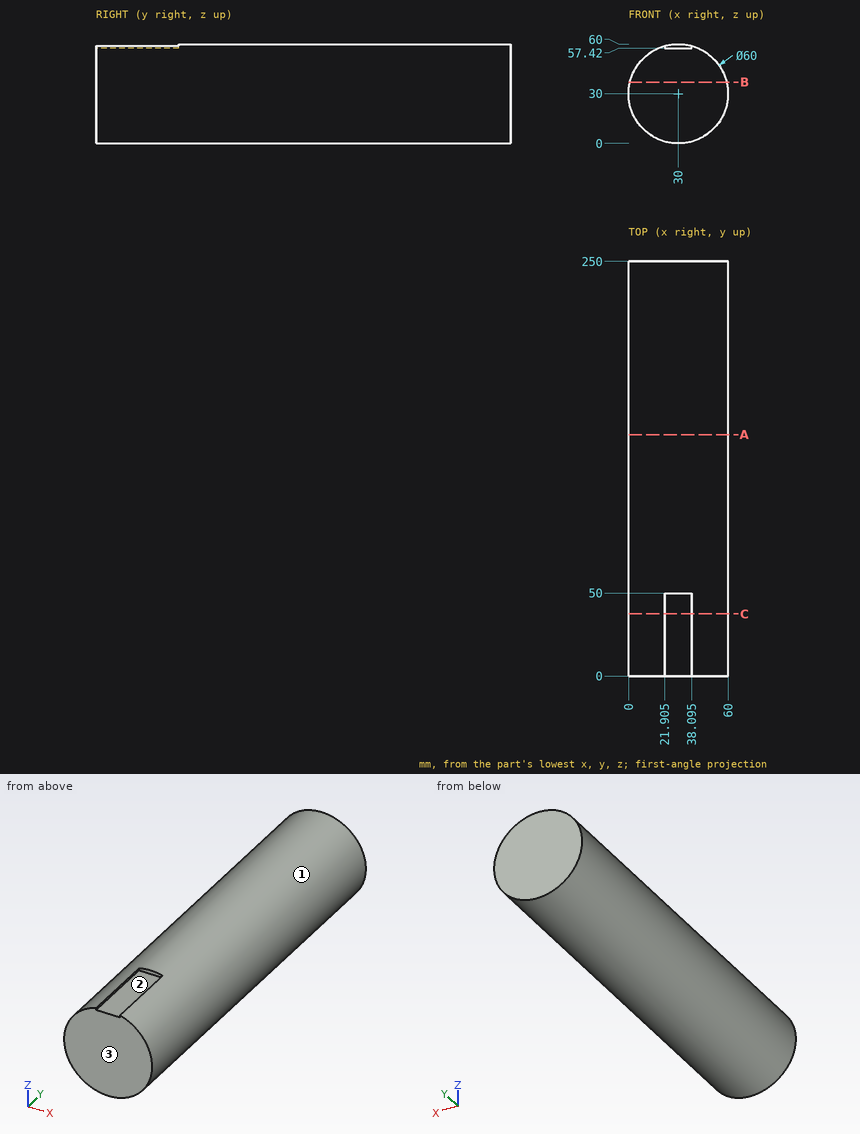
Geometry check sheet. Reference: drawing and pictorial views, mm from the part's lowest x, y, z. Round coordinates to 2 decimals unless told otherwise and drop trailing zeros. Write each loop counter-clockwise with the first axis right and the second up, starting at its lowest first coordinate (ties: lowest second). Pieces come first, ordered by that corner, then holes. Notation, with made-up numbers: (-14.5, 47) -> (27.5, 47) arc R33 cw to (27.5, 75) -> close; hole circle Ø5 at (59, 27). An arc over 180 degrees is marked (long way). One line per question, with ' | ' between items. Start each with the question number.
1. Scan lines: line 1 along X through (y, z) = (144.5, 30); line 2 along X through (y, z) = (219, 54.5) (1 decimal); line 3 along Z through (x, y) = (35.5, 190). Record each from-to range of solid material in increasing order. Write a range as from..to.
2. Sectioned sample at B-B, the plane z = 37. Record the cut outline in (x, y).
3. Sectioned sample at C-C, the plane y = 37.5. Record the cut outline in (x, z) (1 decimal).
4. Depth check by flat-ended pin: pin 1 (5 mm diameter, centred on x = 28.5, y = 16.5, fed in from +Z); pin 2 (8 mm diameter, centred on x = 52.5, z = 46.5, fed in from -Y); pin 3 (1.6 mm diameter, centred on y = 36.5, z = 58, fed in from -X) (1 decimal); pin 4 (4 mm diameter, centred on x = 20, y = 175, fed in from +Z). Enter the tip coordinate at first touch or a pass-through.
5. Release check for a two-part mould opening along X. For the marked faces 1, 2 and 3 record: +X half, -X half, draft (parallel to the pull), parting line (faces both ways), or undercut.
6. Sectioned sample at A-A, the plane y = 145.5. Record the cut outline in (x, z).
Taken from the geometry:
1) line 1: x = 0..60 | line 2: x = 12.7..47.3 | line 3: z = 0.51..59.49
2) outline: (0.83, 0) -> (59.17, 0) -> (59.17, 250) -> (0.83, 250) -> close
3) outline: (21.9, 57.4) -> (21.9, 58.9) arc R30 ccw (long way) to (38.1, 58.9) -> (38.1, 57.4) -> close
4) pin 1: stops at z = 57.42 | pin 2: stops at y = 0 | pin 3: stops at x = 17.3 | pin 4: stops at z = 58.91
5) face 1: parting line | face 2: undercut | face 3: draft
6) outline: circle Ø60 at (30, 30)
